Geometry check sheet. Reference: the model listing, model coordinates, mm. Round coordinates to 2 decimals unless told otherwise and drop trailing zeros. Order: outer loops, then holes, each group sorted by start corner. A loop starts at its lowest first (then second) coordinate and runs counter-clockwise, first axis right, second up. Notation, with made-up numbers: (83, 71.5) - (93, 71.5) arc R26 ccw to (93, 104.5) - close; hole circle Ø9 at (69.5, -20). An arc over 180 degrees is marked (long way). One line per question, with ' | ' between items. Start each with the question number.
Q1. Mould release check, pull along Y, two halves, no side actions. Record for faces 1 (the face through (13.255, 54.828, 1.972)), 2 (the face through (20, 41, 4)), 3 (the face through (20, 0, 2)): +Y half, -Y half, draft (parallel to the pull), parting line (faces both ways), or undercut.
Q2. Material ranges on line 1 along Y through (x, z) = (20, 0.65); line 2 along X through (y, z) = (55, 0.5); line 3 along Y through (x, z) = (21, 0.2), recorded low to high.
Q3. Gauge pin test, flat ends, axial feed: P1, Ø2, axis at x = 21, z = 1, coming from the -Y side; P2, Ø2, axis at x = 6, z = 1.5, coming from the +Y side. Record the tip position at first contact, or that the pin passes through.
Q4. Sectioned sample at C-C, the plane x = 17. Enter the section's corners in (y, z).
Q5. Sectioned sample at D-D, the plane x = 21.5. Enter the section's corners in (y, z).
Q6. Sectioned sample at B-B, the plane z = 1.95. Enter the section's corners in (x, y), then the cut area to 3 significant figures.
Q7. Sectioned sample at A-A, the plane y = 10. Enter the section's corners in (x, z), then the cut area to 3 significant figures.
```python
from build123d import *

# Parameters (mm, degrees)
F0_R     = 2.25
F0_R_2   = 8.5
F1_DEPTH = 4


with BuildPart() as f1:
    # F0 (on Top) → F1 (new body)
    with BuildSketch(Plane.XY):
        with BuildLine():
            Line((0, 60), (0, 0))
            Line((0, 0), (40, 0))
            Line((40, 0), (40, 60))
            ThreePointArc((40, 60), (20, 40), (0, 60))
        make_face()
        with Locations((20, 10)):
            Circle(F0_R, mode=Mode.SUBTRACT)
        with BuildLine():
            ThreePointArc((20, 80), (5.857864, 74.142136), (0, 60))
            ThreePointArc((0, 60), (20, 40), (40, 60))
            ThreePointArc((40, 60), (34.142136, 74.142136), (20, 80))
        make_face()
        with Locations((20, 60)):
            Circle(F0_R_2, mode=Mode.SUBTRACT)
    extrude(amount=F1_DEPTH)


solid = f1.part
```
Determined:
1) face 1: undercut | face 2: draft | face 3: -Y half
2) line 1: y = 0 to 7.75, 12.25 to 51.5, 68.5 to 80 | line 2: x = 0 to 13.13, 26.87 to 40 | line 3: y = 0 to 7.98, 12.02 to 51.56, 68.44 to 79.97
3) P1: stops at y = 0 | P2: stops at y = 75.2
4) outline: (0, 0) - (52.05, 0) - (52.05, 4) - (0, 4) - close; (67.95, 0) - (79.77, 0) - (79.77, 4) - (67.95, 4) - close
5) outline: (0, 0) - (8.32, 0) - (8.32, 4) - (0, 4) - close; (11.68, 0) - (51.63, 0) - (51.63, 4) - (11.68, 4) - close; (68.37, 0) - (79.94, 0) - (79.94, 4) - (68.37, 4) - close
6) outline: (0, 0) - (40, 0) - (40, 60) arc R20 ccw to (20, 80) arc R20 ccw to (0, 60) - close; hole circle Ø17 at (20, 60); hole circle Ø4.5 at (20, 10) | area: 2,790 mm2
7) outline: (0, 0) - (17.75, 0) - (17.75, 4) - (0, 4) - close; (22.25, 0) - (40, 0) - (40, 4) - (22.25, 4) - close | area: 142 mm2
